Source: CAD feature listing. Evaluate the final solid. Frame: model axes, mm. A direction names the side the tool comes from. Give positions to 0.01 mm unless a question says otherwise; leave off trailing zeros. Write each loop counter-clockwise with the first axis right and the second up, starting at its lowest first coordinate (ties: lowest second). Pieces come first, ordered by that corner, then holes. Notation, with made-up numbers: (30, 18) -> (36, 18) arc R18 cw to (36, 25) -> close; hole circle Ø4 at (-34.5, 70.25). An arc over 180 degrees is marked (long way). Use a Markdown table: item, result. Add a question column.
Autodesk Inventor part; units mm, degrees
ref_plane "Start plane" through (0, 0, 0.2121) normal (0, 0, 1) x (1, 0, 0)
ref_plane "End plane" through (0, 0, 480) normal (0, 0, 1) x (1, 0, 0)
ref_plane "Work Plane4" through (0, 12.6061, 0.1061) normal (0, -0.7071, -0.7071) x (1, 0, 0)
ref_plane "Start plane" through (0, 0, 0.2121) normal (0, 0, 1) x (1, 0, 0)
ref_plane "End plane" through (0, 0, 480) normal (0, 0, 1) x (1, 0, 0)
sketch "Sketch" plane through (0, 0, 0) normal (0, 0, 1) x (1, 0, 0)
  line L0 (-12.5, -8.5) -> (-12.5, 8.5)
  line L1 (-8.5, 12.5) -> (8.5, 12.5)
  line L2 (12.5, 8.5) -> (12.5, -8.5)
  line L3 (8.5, -12.5) -> (-8.5, -12.5)
  arc A0 (-12.5, -8.5) -> (-8.5, -12.5) centre (-8.5, -8.5) ccw
  arc A1 (12.5, 8.5) -> (8.5, 12.5) centre (8.5, 8.5) ccw
  arc A2 (-8.5, 12.5) -> (-12.5, 8.5) centre (-8.5, 8.5) ccw
  arc A3 (8.5, -12.5) -> (12.5, -8.5) centre (8.5, -8.5) ccw
  arc A4 (-8.5, 10.5) -> (-10.5, 8.5) centre (-8.5, 8.5) ccw
  line L4 (-8.5, 10.5) -> (8.5, 10.5)
  arc A5 (10.5, 8.5) -> (8.5, 10.5) centre (8.5, 8.5) ccw
  line L5 (10.5, 8.5) -> (10.5, -8.5)
  arc A6 (8.5, -10.5) -> (10.5, -8.5) centre (8.5, -8.5) ccw
  line L6 (8.5, -10.5) -> (-8.5, -10.5)
  arc A7 (-10.5, -8.5) -> (-8.5, -10.5) centre (-8.5, -8.5) ccw
  line L7 (-10.5, -8.5) -> (-10.5, 8.5)
  line L8 (0, 18.6598) -> (0, -18.6598) construction
  line L9 (-18.6598, 0) -> (18.6598, 0) construction
  dimension "d7" = 4
  dimension "d9" = 25
  dimension "d11" = 25
  dimension "d12" = 2
  dimension "d15" = 12.5
  dimension "d16" = 12.5
extrude "Body" add sketch "Sketch" along normal up to surface (479.7879 mm away) from surface at 0.2121
sketch "Sketch3" plane through (0, 0, 0) normal (0, 0, 1) x (1, 0, 0)
  line L0 (0, 0) -> (10, 0)
ref_plane "Work Plane3" through (0, 0, 0) normal (0, -1, 0) x (1, 0, 0)
sketch "Sketch4" plane through (0, 0, 0) normal (0, -1, 0) x (1, 0, 0)
  line L0 (-2, 0.2121) -> (12, 0.2121)
  line L1 (-2, 480) -> (12, 480)
  dimension "d18" = 479.7879
ref_plane "Work Plane4" through (0, 12.6061, 0.1061) normal (0, -0.7071, -0.7071) x (1, 0, 0)
split "Split1" plane through (0, 12.6061, 0.1061) removes the side toward (0, -0.7071, -0.7071)
equation "\"d7\" = G_IR"
equation "\"d9\" = G_W"
equation "\"d11\" = G_H"
equation "\"d12\" = G_T"
equation "\"d15\" = 0.5 * d9"
equation "\"d16\" = 0.5 * d11"
equation "\"d3\" = G_L"
equation "\"G_W\" = 25"
equation "\"G_H\" = 25"
equation "\"G_T\" = 2"
equation "\"G_IR\" = 4"
equation "\"G_L\" = d18"
equation "\"G_OFFSET_START\" = -0.21213"
equation "\"G_OFFSET_END\" = 0"
equation "\"d13\" = -G_OFFSET_START"
properties part number "ISO 4019 - 25x25x2 - 479.788" material "Steel, Mild"
(1) First-contact query: pin 1 Ø4 at (x, y) = (9.5, 9.5) entering from +Z. Flat tip, straight axial feed; report the tip coordinate or a pass-through.
(2) Material intervals for L1, parallel to X at y = 2, z = 277; L2, parallel to X at y = 9.75, z = 263, sorted ascending.
(3) Mould query, pull axis Y, two halves, no side actions, for faces 3 (the flat face through (-11, 0, 480)), 4 (the flat face through (0, -10.5, 248)), 5 (the flat face through (0, -12.5, 249)). Classes: +Y half, -Y half, draft (parallel to the pull), parting line (faces both ways), or undercut.
(4) Cut plane B-B on z = 207. Return the cut outline in (x, y), then the cut area to 3 significant figures.
(5) Cut plane C-C on y = -1.25. Return the cut outline in (x, z), then the cut area to 3 significant figures.
(6) Cut plane A-A on x = 2.5. Return the cut outline in (y, z).
(7) Access query for faces 1 (the flat face through (12.5, 0, 239)), 2 (the flat face through (10.5, 0, 239)). Directions: +Z, -Z, +X, -X, +Y, -Y. A direction counts if a zero-diameter tool reaches every point of the face in a straight line with its end or side. Return the directions, or none.
Output:
| question | item | result |
|---|---|---|
| 1 | pin 1 | z = 480 |
| 2 | L1 | -12.5 to -10.5, 10.5 to 12.5 |
| 2 | L2 | -12.3 to -10.06, 10.06 to 12.3 |
| 3 | face 3 | draft |
| 3 | face 4 | undercut |
| 3 | face 5 | -Y half |
| 4 | outline | (-12.5, -8.5) arc R4 ccw to (-8.5, -12.5) -> (8.5, -12.5) arc R4 ccw to (12.5, -8.5) -> (12.5, 8.5) arc R4 ccw to (8.5, 12.5) -> (-8.5, 12.5) arc R4 ccw to (-12.5, 8.5) -> close; hole (-10.5, -8.5) arc R2 ccw to (-8.5, -10.5) -> (8.5, -10.5) arc R2 ccw to (10.5, -8.5) -> (10.5, 8.5) arc R2 ccw to (8.5, 10.5) -> (-8.5, 10.5) arc R2 ccw to (-10.5, 8.5) -> close |
| 4 | area | 174 mm^2 |
| 5 | outline | (-12.5, 13.96) -> (-10.5, 13.96) -> (-10.5, 480) -> (-12.5, 480) -> close; (10.5, 13.96) -> (12.5, 13.96) -> (12.5, 480) -> (10.5, 480) -> close |
| 5 | area | 1,860 mm^2 |
| 6 | outline | (-12.5, 25.21) -> (-10.5, 23.21) -> (-10.5, 480) -> (-12.5, 480) -> close; (10.5, 2.21) -> (12.5, 0.21) -> (12.5, 480) -> (10.5, 480) -> close |
| 7 | face 1 | +Z, -Z, +X, +Y, -Y |
| 7 | face 2 | +Z, -Z |
